```python
from build123d import *

# Parameters (mm, degrees)
SKETCH1_W           = 469.9
SKETCH1_H           = 292.094
SKETCH1_R           = 2.38125
SKETCH1_W_2         = 52.5
SKETCH1_H_2         = 211.186
BOSS_EXTRUDE1_DEPTH = 10


with BuildPart() as part:
    # Sketch1 → Boss-Extrude1 (new body)
    with BuildSketch(Plane.XY):
        with Locations((213, 105.593)):
            Rectangle(SKETCH1_W, SKETCH1_H)
        with Locations((34.25, -29.180453277)):
            Circle(SKETCH1_R, mode=Mode.SUBTRACT)
        with Locations((70, -29.180453277)):
            Circle(SKETCH1_R, mode=Mode.SUBTRACT)
        with Locations((105.75, -29.180453277)):
            Circle(SKETCH1_R, mode=Mode.SUBTRACT)
        with Locations((141.5, -29.180453277)):
            Circle(SKETCH1_R, mode=Mode.SUBTRACT)
        with Locations((177.25, -29.180453277)):
            Circle(SKETCH1_R, mode=Mode.SUBTRACT)
        with Locations((213, -29.180453277)):
            Circle(SKETCH1_R, mode=Mode.SUBTRACT)
        with Locations((248.75, -29.180453277)):
            Circle(SKETCH1_R, mode=Mode.SUBTRACT)
        with Locations((284.5, -29.180453277)):
            Circle(SKETCH1_R, mode=Mode.SUBTRACT)
        with Locations((320.25, -29.180453277)):
            Circle(SKETCH1_R, mode=Mode.SUBTRACT)
        with Locations((356, -29.180453277)):
            Circle(SKETCH1_R, mode=Mode.SUBTRACT)
        with Locations((391.75, -29.180453277)):
            Circle(SKETCH1_R, mode=Mode.SUBTRACT)
        with Locations((427.5, -29.180453277)):
            Circle(SKETCH1_R, mode=Mode.SUBTRACT)
        with Locations((-1.5, 240.366453277)):
            Circle(SKETCH1_R, mode=Mode.SUBTRACT)
        with Locations((34.25, 240.366453277)):
            Circle(SKETCH1_R, mode=Mode.SUBTRACT)
        with Locations((70, 240.366453277)):
            Circle(SKETCH1_R, mode=Mode.SUBTRACT)
        with Locations((105.75, 240.366453277)):
            Circle(SKETCH1_R, mode=Mode.SUBTRACT)
        with Locations((141.5, 240.366453277)):
            Circle(SKETCH1_R, mode=Mode.SUBTRACT)
        with Locations((177.25, 240.366453277)):
            Circle(SKETCH1_R, mode=Mode.SUBTRACT)
        with Locations((213, 240.366453277)):
            Circle(SKETCH1_R, mode=Mode.SUBTRACT)
        with Locations((-1.5, -29.180453277)):
            Circle(SKETCH1_R, mode=Mode.SUBTRACT)
        with Locations((248.75, 240.366453277)):
            Circle(SKETCH1_R, mode=Mode.SUBTRACT)
        with Locations((284.5, 240.366453277)):
            Circle(SKETCH1_R, mode=Mode.SUBTRACT)
        with Locations((320.25, 240.366453277)):
            Circle(SKETCH1_R, mode=Mode.SUBTRACT)
        with Locations((356, 240.366453277)):
            Circle(SKETCH1_R, mode=Mode.SUBTRACT)
        with Locations((391.75, 240.366453277)):
            Circle(SKETCH1_R, mode=Mode.SUBTRACT)
        with Locations((427.5, 240.366453277)):
            Circle(SKETCH1_R, mode=Mode.SUBTRACT)
        with Locations((34.25, 105.593)):
            Rectangle(SKETCH1_W_2, SKETCH1_H_2, mode=Mode.SUBTRACT)
        with Locations((105.75, 105.593)):
            Rectangle(SKETCH1_W_2, SKETCH1_H_2, mode=Mode.SUBTRACT)
        with Locations((177.25, 105.593)):
            Rectangle(SKETCH1_W_2, SKETCH1_H_2, mode=Mode.SUBTRACT)
        with Locations((248.75, 105.593)):
            Rectangle(SKETCH1_W_2, SKETCH1_H_2, mode=Mode.SUBTRACT)
        with Locations((320.25, 105.593)):
            Rectangle(SKETCH1_W_2, SKETCH1_H_2, mode=Mode.SUBTRACT)
        with Locations((391.75, 105.593)):
            Rectangle(SKETCH1_W_2, SKETCH1_H_2, mode=Mode.SUBTRACT)
    extrude(amount=BOSS_EXTRUDE1_DEPTH)


solid = part.part
```
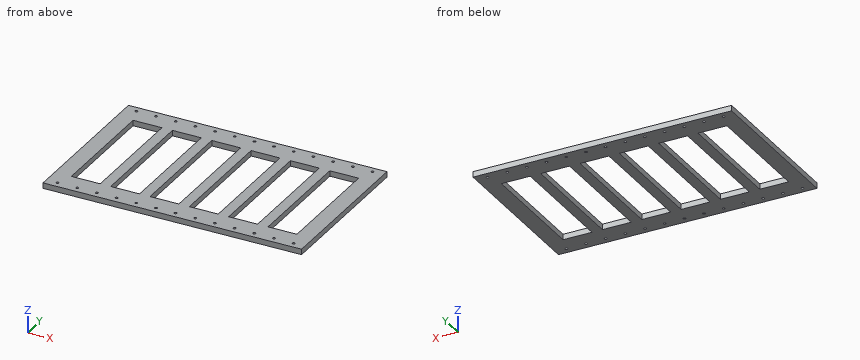
Source: CAD feature listing. Evaluate the final solid. Frame: model axes, mm. Coordinates: 2 decimals unless noted, no trailing zeros. Order: outer loops, then holes, each group sorted by start corner. A loop starts at its lowest first (then second) coordinate and runs counter-clockwise, first axis right, second up. Notation, with made-up numbers: M 0,-16.5 L 36,-16.5 A9 cw 36,-1.5 Z; hole C -12,-2 d5. An arc over 180 degrees is marked long. Write each question's results on one line, items separated by ' | '. Start each with the question number.
1) Line query: line 1 (Y direction, x = 213.5, z = 5.5); line 2 (Y direction, x = 427.5, z = 4); line 3 (Y direction, x = 248.75, z = 3.75). Output: solid intervals per line, ascending. Write a range as from..to.
2) Section query B-B (y = 167.5). Return the cut outline in (x, z).
3) Section query C-C (z = 2.5). Give the number of separate pieces and of enclosed holes in the cut face, plus the area to 3 significant figures.
4) Section query A-A (x = 161). Return the cut outline in (y, z).
5) Contact query for a flat-ended pin moving along its axis: pin 1 Ø4 at (x, y) = (284.5, 240.37) entering from -Z. Output: stop coordinate, or through.
Answers:
1) line 1: y = -40.45..-31.51, -26.85..238.04, 242.69..251.64 | line 2: y = -40.45..-31.56, -26.8..237.99, 242.75..251.64 | line 3: y = -40.45..-31.56, -26.8..0, 211.19..237.99, 242.75..251.64
2) outline: M -21.95,0 L 8,0 L 8,10 L -21.95,10 Z; M 60.5,0 L 79.5,0 L 79.5,10 L 60.5,10 Z; M 132,0 L 151,0 L 151,10 L 132,10 Z; M 203.5,0 L 222.5,0 L 222.5,10 L 203.5,10 Z; M 275,0 L 294,0 L 294,10 L 275,10 Z; M 346.5,0 L 365.5,0 L 365.5,10 L 346.5,10 Z; M 418,0 L 447.95,0 L 447.95,10 L 418,10 Z
3) separate pieces: 1 | enclosed holes: 32 | area: 70,300 mm^2
4) outline: M -40.45,0 L 0,0 L 0,10 L -40.45,10 Z; M 211.19,0 L 251.64,0 L 251.64,10 L 211.19,10 Z
5) pin 1: passes through
